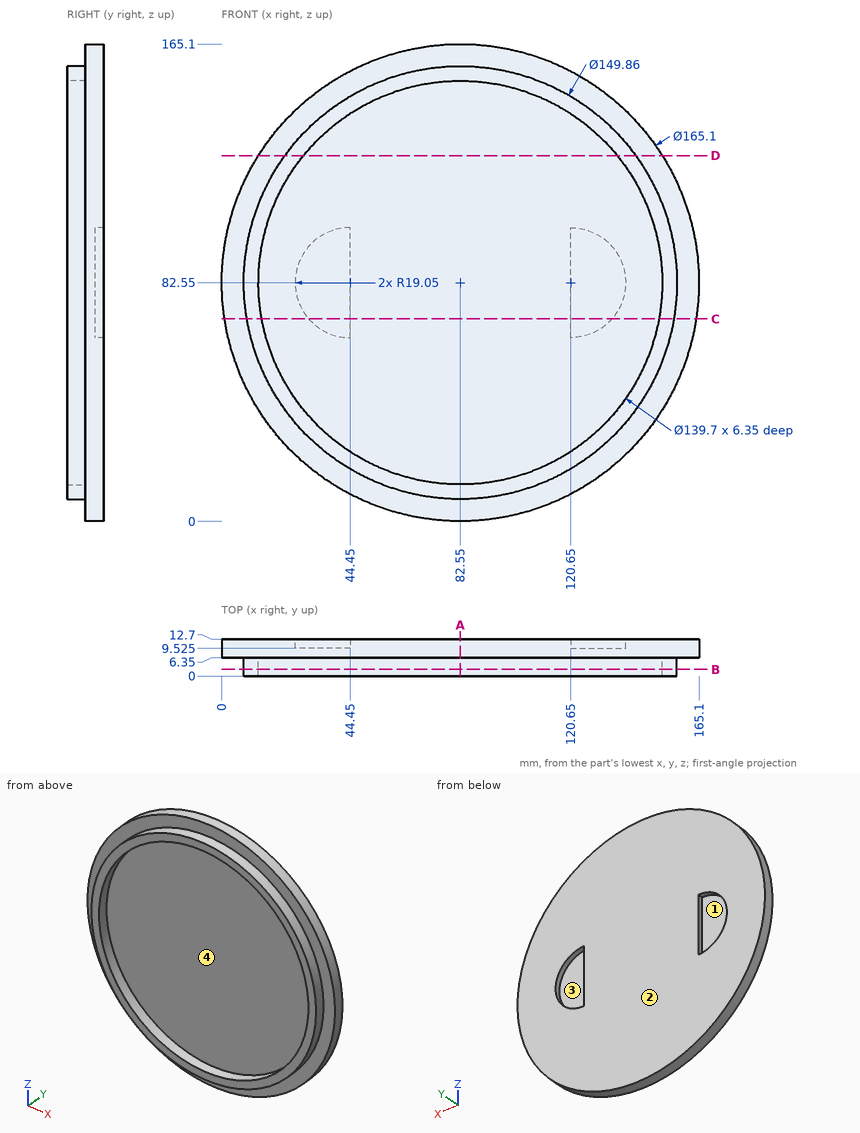
Study the drawing (mm; zero at the part's minimum x, y, z) and answer. A direction names the side the tool comes from. Coordinates: 2 decimals unless noted, no trailing zeros. Write each loop counter-clockwise with the first axis right and the second up, starting at its lowest first coordinate (ties: lowest second). Pieces come first, ordered by that corner, then holes.
Q1. The mould has two halves that part along X. Classify the marked faces 1 and 2: released by +X, released by -X, zero draft, split by the parting line, or undercut.
Returned:
face 1: undercut
face 2: zero draft
Q2. Section C-C, the plane z = 70 is taken. Write down the section's boundary in (x, y) (3 decimals).
Returned:
outline: (0.96, 6.35) - (8.678, 6.35) - (8.678, 0) - (13.837, 0) - (13.837, 6.35) - (151.263, 6.35) - (151.263, 0) - (156.422, 0) - (156.422, 6.35) - (164.14, 6.35) - (164.14, 12.7) - (134.982, 12.7) - (134.982, 9.525) - (120.65, 9.525) - (120.65, 12.7) - (44.45, 12.7) - (44.45, 9.525) - (30.118, 9.525) - (30.118, 12.7) - (0.96, 12.7) - close
Q3. Find the intervals of material crossed by line 1 along X through (y, z) = (3.5, 82.55); line 2 along X through (y, z) = (9.75, 69.5); line 3 along Z through (x, y) = (22, 4.5), in increasing order.
Returned:
line 1: x = 7.62 to 12.7, 152.4 to 157.48
line 2: x = 1.04 to 30.57, 44.45 to 120.65, 134.53 to 164.06
line 3: z = 38.41 to 47.73, 117.37 to 126.69
Q4. Section B-B, the plane y = 2.25 is taken. Write down the section's boundary in (x, z).
Returned:
outline: circle Ø149.86 at (82.55, 82.55); hole circle Ø139.7 at (82.55, 82.55)
Q5. Given P1, Ø2, axis at y = 10, z = 53, coming from the +X side; P2, Ø1.5, axis at y = 10.5, z = 70.5, coming from the +X side; P3, Ø3, axis at y = 4, z = 110.5, coming from the -X side, each flat-ended and moving along its own axis, determine where each tip first touches the part or whether it passes through.
Returned:
P1: stops at x = 160.01
P2: stops at x = 164.32
P3: stops at x = 12.44
Q6. Which of the six approach directions +Z, -Z, +X, -X, +Y, -Y give full straight-line access (tool end or side, diameter ignored) to the marked faces 3 and 4?
Returned:
face 3: +Y
face 4: -Y
Q7. Section A-A, the plane x = 82.55 is taken. Write down the section's boundary in (y, z), then the cut area to 3 significant figures.
Returned:
outline: (0, 7.62) - (6.35, 7.62) - (6.35, 0) - (12.7, 0) - (12.7, 165.1) - (6.35, 165.1) - (6.35, 157.48) - (0, 157.48) - (0, 152.4) - (6.35, 152.4) - (6.35, 12.7) - (0, 12.7) - close
area: 1,110 mm2
Q8. Section D-D, the plane z = 126.5 is taken. Write down the section's boundary in (x, y).
Returned:
outline: (12.67, 6.35) - (21.86, 6.35) - (21.86, 0) - (28.26, 0) - (28.26, 6.35) - (136.84, 6.35) - (136.84, 0) - (143.24, 0) - (143.24, 6.35) - (152.43, 6.35) - (152.43, 12.7) - (12.67, 12.7) - close
